Part model, mm, in its own coordinate system. A direction names the side the tool comes from. Coordinates: 2 decimals unless noted, no trailing zeros. Order: outer loops, then holes, each group sorted by start corner. A loop starts at its lowest first (then second) coordinate and runs counter-clockwise, first axis right, second up.
from build123d import *

# Parameters (mm, degrees)
F0_W      = 127
F0_H      = 50.8
F2_R      = 76.2
F3_DEPTH  = 127
F5_DEPTH  = 76.2
F6_R      = 25.4
F7_R      = 25.4
F8_R      = 12.7
F10_DEPTH = 152.401
F11_R     = 10


with BuildPart() as f1:
    # F0 (on Front) → F1 (revolve)
    with BuildSketch(Plane.XZ):
        with Locations((-92.3652442396, 20.6056353453)):
            Rectangle(F0_W, F0_H)
    revolve(axis=Axis((-155.8652442396, 0, 20.6056353453), (0, 0, -1)))

    # F2 (on face) → F3 (join)
    with BuildSketch(Plane.XY.offset(46.0056353453)):
        with Locations((-155.8652442396, 0)):
            Circle(F2_R)
    extrude(amount=F3_DEPTH)

    # F4 (on face) → F5 (join)
    with BuildSketch(Plane.XY.offset(173.0056353453)):
        Polygon((-130.4652442396, 30.3003561618), (-155.8652442396, 30.3003561618), (-181.2652442396, 30.3003561618), (-181.2652442396, -31.9382007305), (-155.8652442396, -31.9382007305), (-130.4652442396, -31.9382007305), align=None)
    extrude(amount=F5_DEPTH)

    # F6
    f6_edges = [f1.edges().sort_by_distance(p)[0] for p in [
        (-155.865244, 30.300356, 249.205635),
    ]]
    fillet(f6_edges, radius=F6_R)

    # F7
    f7_edges = [f1.edges().sort_by_distance(p)[0] for p in [
        (-155.865244, -31.938201, 249.205635),
    ]]
    fillet(f7_edges, radius=F7_R)

    # F8 (on face) → F10 (cut, through all)
    with BuildSketch(Plane(origin=(-181.2652442396, 0, 0), x_dir=(0, -1, 0), z_dir=(-1, 0, 0))):
        with Locations((0.8146438382, 213.611766696)):
            Circle(F8_R)
    extrude(amount=-F10_DEPTH, mode=Mode.SUBTRACT)

    # F11
    f11_edges = [f1.edges().sort_by_distance(p)[0] for p in [
        (-282.865244, 0, 46.005635),
    ]]
    fillet(f11_edges, radius=F11_R)


solid = f1.part
Q1. Pin check, flat tips, straight feed: pin 1 Ø1 at (y, z) = (16, 33) entering from +X; pin 2 Ø1 at (x, z) = (-127, 121) entering from -Y; pin 3 Ø5 at (y, z) = (61, 118) entering from +X. Stop position of each tip, or through.
Results list:
pin 1: stops at x = -29.81
pin 2: stops at y = -70.72
pin 3: stops at x = -107.04
Q2. Which spindle directions (+Z, -Z, +X, -X, +Y, -Y) get a long thin tool onto all of the face, cutting with end or side? Do faces 5 (the face through (-156, -31.938, 198)), 6 (the face through (-130.465, 6, 202)), 7 (the face through (-156, 30.3, 198)), 8 (the face through (-172.38, -74.39, 108.62)). Say none if no direction does.
Results list:
face 5: +Z, +X, -X, -Y
face 6: +Z, +X, +Y, -Y
face 7: +Z, +X, -X, +Y
face 8: +Z
Q3. Wall check: line 1 along Z through (x, y) = (-199, -4); line 2 along Z through (x, y) = (-118.5, -90.5); line 3 along X through (y, z) = (49.5, 16.5). Give the ranges that are in metal, low to high.
Results list:
line 1: z = -4.79 to 173.01
line 2: z = -4.79 to 46.01
line 3: x = -272.82 to -38.91
Q4. Cut at B-B on z = 64. Write the cut outline in (x, y).
Results list:
outline: circle Ø152.4 at (-155.87, 0)
Q5. Mould opens along Y. For faces 1 (the face through (-156.221, 1.938, 201.214)), 2 (the face through (-155.51, -24.3, 241.96)), 3 (the face through (-181.265, -7, 202)), 4 (the face through (-183.4, 123.98, 15.89)) say: pulls with the +Y half, pulls with the -Y half, needs draft (parallel to the pull), parting line crosses it, or undercut.
Results list:
face 1: undercut
face 2: pulls with the -Y half
face 3: needs draft
face 4: parting line crosses it
Q6. Cut at A-A on y = 0. Write the cut outline in (x, z).
Results list:
outline: (-282.87, -4.79) - (-28.87, -4.79) - (-28.87, 36.01) arc R10 ccw to (-38.87, 46.01) - (-79.67, 46.01) - (-79.67, 173.01) - (-130.47, 173.01) - (-130.47, 200.94) - (-181.27, 200.94) - (-181.27, 173.01) - (-232.07, 173.01) - (-232.07, 46.01) - (-272.87, 46.01) arc R10 ccw to (-282.87, 36.01) - close; (-181.27, 226.29) - (-130.47, 226.29) - (-130.47, 249.21) - (-181.27, 249.21) - close
